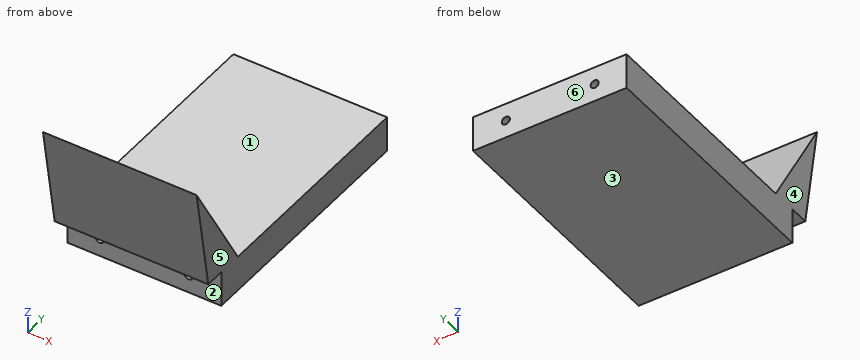
```python
from build123d import *

# Parameters (mm, degrees)
SKETCH1_W                 = 43
SKETCH1_H                 = 10
BOSS_EXTRUDE1_DEPTH       = 70
BOSS_EXTRUDE3_DEPTH       = 43
SKETCH3_R                 = 0.685
CUT_EXTRUDE1_DEPTH        = 15
SKETCH4_R                 = 0.685
CUT_EXTRUDE2_DEPTH        = 15
F_4_40_TAPPED_HOLE1_D     = 2.2606
F_4_40_TAPPED_HOLE1_DEPTH = 7.6
F_4_40_TAPPED_HOLE1_TIP   = 0.679152758
F_4_40_TAPPED_HOLE2_D     = 2.2606
F_4_40_TAPPED_HOLE2_DEPTH = 7.6
F_4_40_TAPPED_HOLE2_TIP   = 0.679152758


with BuildPart() as part:
    # Sketch1 → Boss-Extrude1 (new body)
    with BuildSketch(Plane(origin=(0, 0, 0), x_dir=(1, 0, 0), z_dir=(0, 1, 0))):
        Rectangle(SKETCH1_W, SKETCH1_H)
    extrude(amount=BOSS_EXTRUDE1_DEPTH)

    # Sketch2 → Boss-Extrude3 (add)
    with BuildSketch(Plane(origin=(21.5, 0, 0), x_dir=(0, 0, -1), z_dir=(1, 0, 0))):
        Polygon((-5, 7), (-5, -5.5), (-34.772622472, -10.431034139), align=None)
    extrude(amount=-BOSS_EXTRUDE3_DEPTH)

    # Sketch3 → Cut-Extrude1 (cut)
    with BuildSketch(Plane.XZ):
        with Locations((-12.515, 0)):
            Circle(SKETCH3_R)
        with Locations((12.355, 0)):
            Circle(SKETCH3_R)
    extrude(amount=-CUT_EXTRUDE1_DEPTH, mode=Mode.SUBTRACT)

    # Sketch4 → Cut-Extrude2 (cut)
    with BuildSketch(Plane(origin=(0, 70, 0), x_dir=(1, 0, 0), z_dir=(0, 1, 0))):
        with Locations((-12.565, 0)):
            Circle(SKETCH4_R)
        with Locations((12.305, 0)):
            Circle(SKETCH4_R)
    extrude(amount=-CUT_EXTRUDE2_DEPTH, mode=Mode.SUBTRACT)

    # #4-40 Tapped Hole1
    with Locations(Plane(origin=(0, 70, 0), x_dir=(1, 0, 0), z_dir=(0, 1, 0))):
        with Locations((12.305, 0), (-12.565, 0)):
            Hole(F_4_40_TAPPED_HOLE1_D / 2, depth=F_4_40_TAPPED_HOLE1_DEPTH)
            with Locations((0, 0, -(F_4_40_TAPPED_HOLE1_DEPTH + F_4_40_TAPPED_HOLE1_TIP / 2))):  # 118° drill point
                Cone(0, F_4_40_TAPPED_HOLE1_D / 2, F_4_40_TAPPED_HOLE1_TIP, mode=Mode.SUBTRACT)

    # #4-40 Tapped Hole2
    with Locations(Plane(origin=(0, 0, 0), x_dir=(-1, 0, 0), z_dir=(0, -1, 0))):
        with Locations((-12.355, 0), (12.515, 0)):
            Hole(F_4_40_TAPPED_HOLE2_D / 2, depth=F_4_40_TAPPED_HOLE2_DEPTH)
            with Locations((0, 0, -(F_4_40_TAPPED_HOLE2_DEPTH + F_4_40_TAPPED_HOLE2_TIP / 2))):  # 118° drill point
                Cone(0, F_4_40_TAPPED_HOLE2_D / 2, F_4_40_TAPPED_HOLE2_TIP, mode=Mode.SUBTRACT)


solid = part.part
```
Verification items for the finished model (mm, model axes). Face numbers are marked on the shaded views. A direction names the side the tool comes from. Give positions to 0.01 mm unless a question says otherwise; leave off trailing zeros. Order: outer loops, then holes, each group sorted by start corner. A loop starts at its lowest first (then second) coordinate and runs counter-clockwise, first axis right, second up. Notation, with made-up numbers: M 86.25,28 L 117.25,28 A14 cw 117.25,32 Z; hole C 15.25,-31.75 d7. An arc over 180 degrees is marked long. Answer in a Markdown table with one row per item. Add a question column.
Item 1: Gauge pin test, flat ends, axial feed: pin 1 (11 mm diameter, centred on x = -3, z = 0, fed in from -Y); pin 2 (2 mm diameter, centred on x = 12.355, z = 0, fed in from -Y); pin 3 (1.2 mm diameter, centred on x = -12.515, z = 0, fed in from +Y); pin 4 (6 mm diameter, centred on y = -0.5, z = 26, fed in from +X). Record the tip position at first contact, or that the pin passes through.
Item 2: Scan lines: probe 1 along X at (y, z) = (59.75, 0); probe 2 along Z at (x, y) = (-0.5, 54); probe 3 along Y at (x, z) = (-14, 1). Record each from-to range of solid material in increasing order. Write a range as from..to.
Item 3: Section check C-C, the plane z = -3. Enter the section's corners in (x, y), and give its area (3 significant figures).
Item 4: Tool access check on the marked faces 1, 2 and 3. Record the directions out of +Z, -Z, +X, -X, +Y, -Y that give a thin tool (end or side, any length) a straight path to the whole face; none if there is none.
Item 5: Section check B-B, the plane y = 12. Enter the section's corners in (x, z) (3 decimals).
Item 6: Section check D-D, the plane y = 45. Enter the section's corners in (x, z).
Item 7: Section check A-A, the plane x = -19. Enter the section's corners in (y, z).
Item 8: Mould release check, pull along X, two halves, no side actions. Record for the marked faces 4, 5 and 6: released by +X, released by -X, zero draft, split by the parting line, or undercut.
Filled sheet:
| question | item | result |
|---|---|---|
| 1 | pin 1 | stops at y = -5.58 |
| 1 | pin 2 | stops at y = 7.68 |
| 1 | pin 3 | stops at y = 55 |
| 1 | pin 4 | passes through |
| 2 | probe 1 | x = -21.5..-13.25, -11.88..11.62, 12.99..21.5 |
| 2 | probe 2 | z = -5..5 |
| 2 | probe 3 | y = 0..70 |
| 3 | outline | M -21.5,0 L 21.5,0 L 21.5,70 L -21.5,70 Z |
| 3 | area | 3,010 mm^2 |
| 4 | face 1 | +Z, +X, -X, +Y |
| 4 | face 2 | -Z, +X, -X, -Y |
| 4 | face 3 | -Z, +X, -X, +Y, -Y |
| 5 | outline | M -21.5,-5 L 21.5,-5 L 21.5,5 L -21.5,5 Z; hole C -12.515,0 d1.37; hole C 12.355,0 d1.37 |
| 6 | outline | M -21.5,-5 L 21.5,-5 L 21.5,5 L -21.5,5 Z |
| 7 | outline | M -10.43,34.77 L -5.5,5 L 0,5 L 0,-5 L 70,-5 L 70,5 L 7,5 Z |
| 8 | face 4 | released by -X |
| 8 | face 5 | released by +X |
| 8 | face 6 | zero draft |
